Autodesk Inventor part; units mm, degrees
ref_plane "YZ Plane" through (0, 0, 0) normal (1, 0, 0) x (0, 1, 0)
ref_plane "XZ Plane" through (0, 0, 0) normal (0, 1, 0) x (-1, 0, 0)
ref_plane "XY Plane" through (0, 0, 0) normal (0, 0, 1) x (1, 0, 0)
sketch "Sketch1" plane through (0, 0, 0) normal (0, 1, 0) x (-1, 0, 0)
  line L0 (0, 0) -> (0, -135)
  line L1 (0, -135) -> (73.0002, -135)
  line L2 (73.0002, -135) -> (73.0002, 0)
  circle A0 centre (3, -3) radius 1.75
  line L3 (73.0002, 0) -> (0, 0)
  circle A1 centre (70.0002, -3) radius 1.75
  circle A2 centre (70.0002, -132) radius 1.75
  circle A3 centre (3, -132) radius 1.75
  circle A4 centre (13, -131) radius 0.75
  circle A5 centre (19.5, -131) radius 0.75
  circle A6 centre (26, -131) radius 0.75
  circle A7 centre (32.5, -131) radius 0.75
  circle A8 centre (39, -131) radius 0.75
  circle A9 centre (45.5, -131) radius 0.75
  circle A10 centre (52, -131) radius 0.75
  circle A11 centre (58.5, -131) radius 0.75
  circle A12 centre (11, -3) radius 0.55
  circle A13 centre (11, -5.54) radius 0.55
  circle A14 centre (11, -8.08) radius 0.55
  circle A15 centre (11, -10.62) radius 0.55
  circle A16 centre (60.0002, -5) radius 0.75
  circle A17 centre (60.0002, -11.5) radius 0.75
  circle A18 centre (60.0002, -18) radius 0.75
  circle A19 centre (60.0002, -24.5) radius 0.75
  circle A20 centre (60.0002, -31) radius 0.75
  circle A21 centre (60.0002, -37.5) radius 0.75
  circle A22 centre (60.0002, -44) radius 0.75
  circle A23 centre (60.0002, -50.5) radius 0.75
  line L4 (47, -21) -> (26, -21) construction
  line L5 (44, -53) -> (23, -53) construction
  line L6 (47, -85) -> (26, -85) construction
  line L7 (50, -115) -> (29, -115) construction
  line L8 (47, -21) -> (47, -11.5) construction
  line L9 (26, -21) -> (26, -11.5) construction
  line L10 (44, -53) -> (44, -43.5) construction
  line L11 (23, -53) -> (23, -43.5) construction
  line L12 (26, -85) -> (26, -75.5) construction
  line L13 (47, -85) -> (47, -75.5) construction
  line L14 (50, -115) -> (50, -105.5) construction
  line L15 (29, -115) -> (29, -105.5) construction
  circle A24 centre (29, -105.5) radius 0.45
  circle A25 centre (50, -105.5) radius 0.45
  circle A26 centre (47, -75.5) radius 0.45
  circle A27 centre (26, -75.5) radius 0.45
  circle A28 centre (44, -43.5) radius 0.45
  circle A29 centre (23, -43.5) radius 0.45
  circle A30 centre (26, -11.5) radius 0.45
  circle A31 centre (47, -11.5) radius 0.45
  dimension "d42" = 3.5
  dimension "d52" = 3
  dimension "d53" = 3
  dimension "d54" = 135
  dimension "d55" = 73.0002
  dimension "d56" = 3.5
  dimension "d57" = 3.5
  dimension "d58" = 3.5
  dimension "d59" = 3
  dimension "d60" = 3
  dimension "d61" = 3
  dimension "d62" = 3
  dimension "d63" = 3
  dimension "d64" = 3
  dimension "d65" = 1.5
  dimension "d66" = 4
  dimension "d67" = 13
  dimension "d70" = 6.5
  dimension "d75" = 1.1
  dimension "d76" = 3
  dimension "d77" = 11
  dimension "d80" = 2.54
  dimension "d85" = 1.5
  dimension "d86" = 13
  dimension "d87" = 5
  dimension "d90" = 6.5
  dimension "d95" = 21
  dimension "d96" = 21
  dimension "d97" = 21
  dimension "d98" = 21
  dimension "d99" = 26
  dimension "d100" = 114
  dimension "d101" = 23
  dimension "d102" = 82
  dimension "d103" = 26
  dimension "d104" = 50
  dimension "d105" = 29
  dimension "d106" = 20
  dimension "d115" = 0.9
  dimension "d128" = 0.9
  dimension "d141" = 0.9
  dimension "d154" = 0.9
  dimension "d167" = 0.9
  dimension "d180" = 0.9
  dimension "d193" = 0.9
  dimension "d206" = 0.9
  dimension "d209" = 9.5
  dimension "d210" = 9.5
  dimension "d211" = 9.5
  dimension "d212" = 9.5
  dimension "d213" = 9.5
  dimension "d214" = 9.5
  dimension "d215" = 9.5
  dimension "d216" = 9.5
extrude "Extrusion1" add sketch "Sketch1" along normal blind 1.6
sketch "Sketch2" plane through (0, 0, 0) normal (0, -1, 0) x (1, 0, 0)
  circle A0 centre (-60.0002, -5) radius 0.75 construction
  circle A1 centre (-60.0002, -11.5) radius 0.75 construction
  circle A2 centre (-60.0002, -18) radius 0.75 construction
  circle A3 centre (-60.0002, -24.5) radius 0.75 construction
  circle A4 centre (-60.0002, -31) radius 0.75 construction
  circle A5 centre (-11, -3) radius 0.55 construction
  circle A6 centre (-11, -5.54) radius 0.55 construction
  circle A7 centre (-11, -8.08) radius 0.55 construction
  circle A8 centre (-11, -10.62) radius 0.55 construction
  circle A9 centre (-60.0002, -37.5) radius 0.75 construction
  circle A10 centre (-60.0002, -44) radius 0.75 construction
  circle A11 centre (-60.0002, -50.5) radius 0.75 construction
  circle A12 centre (-58.5, -131) radius 0.75 construction
  circle A13 centre (-52, -131) radius 0.75 construction
  circle A14 centre (-45.5, -131) radius 0.75 construction
  circle A15 centre (-39, -131) radius 0.75 construction
  circle A16 centre (-26, -131) radius 0.75 construction
  circle A17 centre (-19.5, -131) radius 0.75 construction
  circle A18 centre (-13, -131) radius 0.75 construction
  circle A19 centre (-32.5, -131) radius 0.75 construction
  circle A20 centre (-60.0002, -31) radius 0.75 construction
  circle A21 centre (-60.0002, -24.5) radius 0.75 construction
  circle A22 centre (-60.0002, -11.5) radius 0.75
  point P0 (0, 0)
properties part number "powerDistributionPCB" material "GFRP"
Check sheet for the modelled part. Datum: model origin and axes. Units: mm. Round coordinates to 2 decimals unless told otherwise and drop trailing zeros. Order: outer loops, then holes, each group sorted by start corner. A loop starts at its lowest first (then second) coordinate and runs counter-clockwise, first axis right, second up.
Q1. Draft check along X on faces 1 (the face through (-69.62, 0.79, -130.29)), 2 (the face through (-3.81, 0.79, -130.45)), 3 (the face through (-36, 1.6, -67)). Enter one of: pulls with the +X half, pulls with the -X half, needs draft (parallel to the pull), parting line crosses it, or undercut.
Filled sheet:
face 1: undercut
face 2: undercut
face 3: needs draft
Q2. Scan lines: L1, parallel to Z at x = -47, y = 1.1; L2, parallel to Z at x = -11, y = 1.25; L3, parallel to X at y = 1.1, z = -75.5. Record each from-to range of solid material in increasing order.
Filled sheet:
L1: z = -135 to -75.95, -75.05 to -11.95, -11.05 to 0
L2: z = -135 to -11.17, -10.07 to -8.63, -7.53 to -6.09, -4.99 to -3.55, -2.45 to 0
L3: x = -73 to -47.45, -46.55 to -26.45, -25.55 to 0
Q3. Cross-section at A-A, the plane x = -3. Enter the section's corners in (y, z).
Filled sheet:
outline: (0, -135) - (1.6, -135) - (1.6, -133.75) - (0, -133.75) - close; (0, -130.25) - (1.6, -130.25) - (1.6, -4.75) - (0, -4.75) - close; (0, -1.25) - (1.6, -1.25) - (1.6, 0) - (0, 0) - close
